The listing builds one solid part. Answer for the finished solid, in the listing's coordinates (mm). A direction names the side the tool comes from. Give positions to 0.01 mm unless a question says otherwise; leave off trailing zeros. Loops run counter-clockwise (first coordinate to the right, second up) from the corner with the lowest first, then second, coordinate; pieces in that order, holes last. Notation, with made-up numbers: M 82,-31 L 93,-31 A15 ccw 93,-24 Z; hole C 81.5,83 d2. An arc over 180 degrees is marked long. Use one line per item in the form item = value. Start each with the question number.
1. Straight lines are drawn through the part: line 1 (X direction, y = 57.5, z = 8.75); line 2 (X direction, y = 9.5, z = 6.5); line 3 (Y direction, x = -17, z = 9.5). For each, find the intervals that lie inside material, in ascending order. Write a range as from..to.
2. The part is cut by section C-C (y = 36). Write down the section's boundary in (x, z), and give its area (3 significant figures).
3. The part is cut by section D-D (x = -1). Write down the section's boundary in (y, z).
4. The mould has two halves that part along X. Classify faces 5 (the face through (3.088, 48, 6)), 6 (the face through (-8.331, 31.457, 6.499)), 7 (the face through (-22.48, -0.9, 6.11)): released by +X, released by -X, zero draft, split by the parting line, or undercut.
5. For faces 1 (the face through (15, 4, 6.35)), 2 (the face through (14.724, 2.862, 3.131)), 3 (the face through (22.45, -1.5, 6.11)), 4 (the face through (-5.13, 15.99, 3.13)), determine the directions among +Z, -Z, +X, -X, +Y, -Y from which every point of the face is accessible in a straight line to the end or side of a thin tool.
6. Each of these flat-tipped pins is pushed along its axis until it touches: pin 1 Ø6 at (y, z) = (30, 4.5) entering from +X; pin 2 Ø6 at (y, z) = (63.5, 4) entering from -X; pin 3 Ø1.5 at (x, z) = (-17, 7.5) entering from +Y. Where does it stop, or does it pass through?
7. The part is cut by section B-B (z = 1.5). Write down the section's boundary in (x, y), and give its area (3 significant figures).
8. The part is cut by section A-A (y = 62). Write down the section's boundary in (x, z), and give its area (3 significant figures).
from build123d import *

# Parameters (mm, degrees)
F1_DEPTH = 12.7
F2_DEPTH = 6.35
F4_D     = 6.7564
F5_R     = 5.08


with BuildPart() as f1:
    # F0 (on Top) → F1 (new body)
    with BuildSketch(Plane.XY):
        with BuildLine():
            Line((-13.9034517987, 76.1113017797), (-13.9034517987, 17.6902240822))
            ThreePointArc((-13.9034517987, 17.6902240822), (-22.46786683, -1.2020649347), (-11.9365793678, -19.0727049208))
            Line((-11.9365793678, -19.0727049208), (-10.045198296, -16.337374341))
            ThreePointArc((-10.045198296, -16.337374341), (-18.7984085357, 3.7994270212), (-2.9118661168, 18.9561822338))
            Line((-2.9118661168, 18.9561822338), (-2.9118661168, 77.1448761225))
            Line((-2.9118661168, 77.1448761225), (3.0881338832, 77.1448761225))
            Line((3.0881338832, 77.1448761225), (3.0881338832, 18.928265591))
            ThreePointArc((3.0881338832, 18.928265591), (18.8158827453, 3.7119221002), (10.045198296, -16.337374341))
            Line((10.045198296, -16.337374341), (11.9365793678, -19.0727049208))
            ThreePointArc((11.9365793678, -19.0727049208), (22.46786683, -1.2020649347), (13.9034517987, 17.6902240822))
            Line((13.9034517987, 17.6902240822), (13.9034517987, 76.9488066435))
            Line((13.9034517987, 76.9488066435), (13.9034517987, 77.005261239))
            ThreePointArc((13.9034517987, 77.005261239), (0.4055063748, 90.8876688225), (-13.9034517987, 77.8427661028))
            Line((-13.9034517987, 77.8427661028), (-13.9034517987, 76.1113017797))
        make_face()
    extrude(amount=F1_DEPTH)

    # F0 (on Top) → F2 (join)
    with BuildSketch(Plane.XY):
        with BuildLine():
            Line((-13.9034517987, 76.1113017797), (-13.9034517987, 17.6902240822))
            ThreePointArc((-13.9034517987, 17.6902240822), (-22.46786683, -1.2020649347), (-11.9365793678, -19.0727049208))
            Line((-11.9365793678, -19.0727049208), (-10.045198296, -16.337374341))
            ThreePointArc((-10.045198296, -16.337374341), (-18.7984085357, 3.7994270212), (-2.9118661168, 18.9561822338))
            Line((-2.9118661168, 18.9561822338), (-2.9118661168, 77.1448761225))
            Line((-2.9118661168, 77.1448761225), (3.0881338832, 77.1448761225))
            Line((3.0881338832, 77.1448761225), (3.0881338832, 18.928265591))
            ThreePointArc((3.0881338832, 18.928265591), (18.8158827453, 3.7119221002), (10.045198296, -16.337374341))
            Line((10.045198296, -16.337374341), (11.9365793678, -19.0727049208))
            ThreePointArc((11.9365793678, -19.0727049208), (22.46786683, -1.2020649347), (13.9034517987, 17.6902240822))
            Line((13.9034517987, 17.6902240822), (13.9034517987, 76.9488066435))
            Line((13.9034517987, 76.9488066435), (13.9034517987, 77.005261239))
            ThreePointArc((13.9034517987, 77.005261239), (0.4055063748, 90.8876688225), (-13.9034517987, 77.8427661028))
            Line((-13.9034517987, 77.8427661028), (-13.9034517987, 76.1113017797))
        make_face()
        with BuildLine():
            ThreePointArc((-13.9034517987, 77.8427661028), (-13.9304052278, 76.9770339413), (-13.9034517987, 76.1113017797))
            Line((-13.9034517987, 76.1113017797), (-13.9034517987, 77.8427661028))
        make_face()
        with BuildLine():
            ThreePointArc((-2.9118661168, 18.9561822338), (-18.7984085357, 3.7994270212), (-10.045198296, -16.337374341))
            Line((-10.045198296, -16.337374341), (-9.8947915389, -13.8333481617))
            Line((-9.8947915389, -13.8333481617), (-11.5102852396, -9.6183851921))
            ThreePointArc((-11.5102852396, -9.6183851921), (-14.7467682956, 2.7445992121), (-7.2791813889, 13.1153924191))
            Line((-7.2791813889, 13.1153924191), (-2.9118661168, 18.9561822338))
        make_face()
        with BuildLine():
            ThreePointArc((10.045198296, -16.337374341), (18.8158827453, 3.7119221002), (3.0881338832, 18.928265591))
            Line((3.0881338832, 18.928265591), (7.3907075504, 13.0528710215))
            ThreePointArc((7.3907075504, 13.0528710215), (14.758331433, 2.6817258086), (11.5102852396, -9.6183851921))
            Line((11.5102852396, -9.6183851921), (9.8947915389, -13.8333481617))
            Line((9.8947915389, -13.8333481617), (9.9547252954, -16.3926585232))
            ThreePointArc((9.9547252954, -16.3926585232), (10, -16.3650789538), (10.045198296, -16.337374341))
        make_face()
    extrude(amount=F2_DEPTH)

    # F4 (through all)
    with Locations(Plane(origin=(-13.9034517987, 0, 0), x_dir=(0, -1, 0), z_dir=(-1, 0, 0))):
        with Locations((-34.83145684, 6.35)):
            Hole(F4_D / 2)

    # F5
    f5_edges = [f1.edges().sort_by_distance(p)[0] for p in [
        (-18.798409, 3.799427, 12.7),
        (18.815883, 3.711922, 12.7),
    ]]
    fillet(f5_edges, radius=F5_R)


solid = f1.part
Derived:
q1.line_1 = -13.9..-2.91, 3.09..13.9
q1.line_2 = -20.4..-16.66, 16.66..20.4
q1.line_3 = -14.74..-9.63, 9.63..14.74
q2.outline = M -13.9,0 L -2.91,0 L -2.91,3.18 L -13.9,3.18 Z; M -13.9,9.52 L -2.91,9.52 L -2.91,12.7 L -13.9,12.7 Z; M 3.09,0 L 13.9,0 L 13.9,3.18 L 3.09,3.18 Z; M 3.09,9.52 L 13.9,9.52 L 13.9,12.7 L 3.09,12.7 Z
q2.area = 139 mm2
q3.outline = M 77.14,0 L 90.86,0 L 90.86,12.7 L 77.14,12.7 Z
q4.face_5 = undercut
q4.face_6 = zero draft
q4.face_7 = released by -X
q5.face_1 = +Z
q5.face_2 = +Z, -Z
q5.face_3 = +Z, -Z, +X
q5.face_4 = +Z, -Z, -Y
q6.pin_1 = 13.9
q6.pin_2 = -13.9
q6.pin_3 = 15.56
q7.outline = M -13.9,17.69 A22.5 ccw -11.94,-19.07 L -10.05,-16.34 L -9.89,-13.83 L -11.51,-9.62 A15 cw -7.28,13.12 L -2.91,18.96 L -2.91,77.14 L 3.09,77.14 L 3.09,18.93 L 7.39,13.05 A15 cw 11.51,-9.62 L 9.89,-13.83 L 9.95,-16.39 A19.18 ccw 10.05,-16.34 L 11.94,-19.07 A22.5 ccw 13.9,17.69 L 13.9,77.01 A13.92 ccw long -13.9,76.11 Z
q7.area = 2,180 mm2
q8.outline = M -13.9,0 L -2.91,0 L -2.91,12.7 L -13.9,12.7 Z; M 3.09,0 L 13.9,0 L 13.9,12.7 L 3.09,12.7 Z
q8.area = 277 mm2
